Part model, mm, in its own coordinate system. A direction names the side the tool comes from. Give positions to 0.01 mm unless a question says otherwise; leave off trailing zeros. Loops run counter-clockwise (first coordinate to the right, second up) from the corner with the lowest first, then second, coordinate; pieces in that order, holes last. Notation, with made-up numbers: (40, 8) -> (67, 8) arc R6 cw to (67, 19) -> close; hole circle Ø6 at (3.25, 10.5). An arc over 180 degrees is marked (long way). One line per question, with ' | ' between items.
```python
from build123d import *
from build123d.topology import SkipClean

# Parameters (mm, degrees)
AUFSATZ_LINEAR_AUSTRAGEN1_DEPTH = 4
SKIZZE2_R                       = 3
AUFSATZ_LINEAR_AUSTRAGEN2_DEPTH = 20
AUFSATZ_LINEAR_START            = -3
AUFSATZ_LINEAR_AUSTRAGEN3_DEPTH = 3
AUFSATZ_LINEAR_START_2          = -4
SKIZZE4_R                       = 3
AUFSATZ_LINEAR_AUSTRAGEN4_DEPTH = 5
SKIZZE5_R                       = 1.7
SCHNITT_LINEAR_AUSTRAGEN1_DEPTH = 4


with BuildPart() as part:
    # Skizze1 → Aufsatz-Linear austragen1 (new body)
    with BuildSketch(Plane.XY):
        with BuildLine():
            Line((43.5, -13.943887949), (43.5, -46.908717461))
            ThreePointArc((43.5, -46.908717461), (40.5, -49.908717461), (37.5, -46.908717461))
            Line((37.5, -46.908717461), (37.5, -13.943887949))
            ThreePointArc((37.5, -13.943887949), (40.5, -10.943887949), (43.5, -13.943887949))
        make_face()
    extrude(amount=AUFSATZ_LINEAR_AUSTRAGEN1_DEPTH)

    # Skizze2 → Aufsatz-Linear austragen2 (add)
    with SkipClean():  # the faces are left unmerged after this step: merging them gives an invalid solid
        with BuildSketch(Plane.XY.offset(4)):
            with Locations((40.5, -13.943887949)):
                Circle(SKIZZE2_R)
            with Locations(Location((40.5, -36.443887949, 0), (0, 0, 180))):
                Circle(SKIZZE2_R)
        extrude(amount=AUFSATZ_LINEAR_AUSTRAGEN2_DEPTH)
    add(part.part.scale(1), mode=Mode.REPLACE)  # the faces are merged on a copy

    # Skizze3 → Aufsatz-Linear austragen3 (add)
    with BuildSketch(Plane.XY.offset(24).offset(AUFSATZ_LINEAR_START)):
        with BuildLine():
            Line((43.5, -13.943887949), (43.5, -36.443887949))
            ThreePointArc((43.5, -36.443887949), (40.5, -39.443887949), (37.5, -36.443887949))
            Line((37.5, -36.443887949), (37.5, -13.943887949))
            ThreePointArc((37.5, -13.943887949), (40.5, -10.943887949), (43.5, -13.943887949))
        make_face()
    extrude(amount=AUFSATZ_LINEAR_AUSTRAGEN3_DEPTH)

    # Skizze4 → Aufsatz-Linear austragen4 (add)
    with BuildSketch(Plane.XY.offset(4).offset(AUFSATZ_LINEAR_START_2)):
        with Locations((40.5, -46.908717461)):
            Circle(SKIZZE4_R)
    extrude(amount=AUFSATZ_LINEAR_AUSTRAGEN4_DEPTH)

    # Skizze5 → Schnitt-Linear austragen1 (cut)
    with BuildSketch(Plane(origin=(0, 0, 0), x_dir=(-1, 0, 0), z_dir=(0, 0, -1))):
        with Locations((-40.5, -13.943887949)):
            Circle(SKIZZE5_R)
        with Locations(Location((-40.5, -46.908717461, 0), (0, 0, 180))):
            Circle(SKIZZE5_R)
    extrude(amount=-SCHNITT_LINEAR_AUSTRAGEN1_DEPTH, mode=Mode.SUBTRACT)


solid = part.part
```
1) Saw through at B-B (z = 3.5). Give the cut face in (x, y), and give its area (3 significant figures).
Found:
outline: (37.5, -46.91) arc R3 ccw to (43.5, -46.91) -> (43.5, -13.94) arc R3 ccw to (37.5, -13.94) -> close; hole circle Ø3.4 at (40.5, -46.91); hole circle Ø3.4 at (40.5, -13.94) | area: 208 mm2
2) Saw through at D-D (z = 13). Give the cut face in (x, y), and give its area (3 significant figures).
Found:
outline: circle Ø6 at (40.5, -36.44); circle Ø6 at (40.5, -13.94) | area: 56.5 mm2
3) Tool access for faces 1 (the flat face through (37.5, -25, 22)), 2 (the flat face through (40, -47, 5)), 3 (the cylindrical face through (41.75, -12.79, 1.97)), 4 (the flat face through (41, -42, 4)): list every direction of +Z, -Z, +X, -X, +Y, -Y with a clear straight run to the whole face (end or side of a thin tool).
Found:
face 1: +Z, -Z, -X, +Y, -Y | face 2: +Z, +X, -X, -Y | face 3: -Z | face 4: +Z
4) Pull direction Z, two halves, no side cores. Call faces 5 (the flat face through (41, -14, 4)), 6 (the flat face through (41, -25, 4)), 7 (the flat face through (43.5, -25, 22)): pulls with the +Z half, pulls with the -Z half, needs draft (parallel to the pull), parting line crosses it, or undercut.
Found:
face 5: pulls with the -Z half | face 6: undercut | face 7: needs draft
5) Drill centre lines: line 1 (Z direction, x = 40, y = -28); line 2 (Y direction, x = 41.3, z = 2.75); line 3 (Z direction, x = 38.65, y = -48). Where is each one in solid material? Low to high.
Found:
line 1: 0 to 4, 21 to 24 | line 2: -49.8 to -48.41, -45.41 to -15.44, -12.44 to -11.05 | line 3: 0 to 5
6) Saw through at A-A (y = -30). Give the cut face in (x, z), and give its area (3 significant figures).
Found:
outline: (37.5, 0) -> (43.5, 0) -> (43.5, 4) -> (37.5, 4) -> close; (37.5, 21) -> (43.5, 21) -> (43.5, 24) -> (37.5, 24) -> close | area: 42.0 mm2
7) Pin check, flat tips, straight feed: P1, Ø2.5, axis at x = 40, y = -14, coming from the -Z side; P2, Ø2, axis at x = 40.5, y = -13.94, coming from the -Z side; P3, Ø5, axis at y = -42.5, z = 21.5, coming from the -X side. Stop position of each tip, or through.
Found:
P1: z = 0 | P2: z = 4 | P3: through
8) Saw through at C-C (x = 40.5). Give the cut face in (y, z), and give its area (3 significant figures).
Found:
outline: (-49.91, 0) -> (-48.61, 0) -> (-48.61, 4) -> (-45.21, 4) -> (-45.21, 0) -> (-15.64, 0) -> (-15.64, 4) -> (-12.24, 4) -> (-12.24, 0) -> (-10.94, 0) -> (-10.94, 24) -> (-39.44, 24) -> (-39.44, 4) -> (-43.91, 4) -> (-43.91, 5) -> (-49.91, 5) -> close; hole (-33.44, 4) -> (-16.94, 4) -> (-16.94, 21) -> (-33.44, 21) -> close | area: 424 mm2
